Could you check a few things on this model? Use its own coordinates, in mm. A direction names the side the tool comes from. Coordinates: 2 decimals unless noted, no trailing zeros. Loops run counter-clockwise (first coordinate to the right, second up) from the corner with the lowest first, then second, coordinate; pieces in that order, holes last.
from build123d import *

# Parameters (mm, degrees)
SKETCH_1_R          = 12.5
EXTRUDE_3_DEPTH     = 30
SKETCH_3_R          = 1.5
CUT_EXTRUDE_1_DEPTH = 15
SKETCH_4_R          = 6
EXTRUDE_4_DEPTH     = 2
SKETCH_5_R          = 2
EXTRUDE_5_DEPTH     = 10


with BuildPart() as part:
    # 草图1 → 凸台-拉伸3 (new body)
    with BuildSketch(Plane.XY):
        Circle(SKETCH_1_R)
    extrude(amount=EXTRUDE_3_DEPTH)

    # 草图3 → 切除-拉伸1 (cut)
    with BuildSketch(Plane(origin=(0, 0, 0), x_dir=(-1, 0, 0), z_dir=(0, 0, -1))):
        with Locations((8.5, 0)):
            Circle(SKETCH_3_R)
        with Locations((-8.5, 0)):
            Circle(SKETCH_3_R)
    extrude(amount=-CUT_EXTRUDE_1_DEPTH, mode=Mode.SUBTRACT)

    # 草图4 → 凸台-拉伸4 (add)
    with BuildSketch(Plane(origin=(0, 0, 0), x_dir=(-1, 0, 0), z_dir=(0, 0, -1))):
        with Locations(Location((0, 0, 0), (0, 0, 180))):
            Circle(SKETCH_4_R)
    extrude(amount=EXTRUDE_4_DEPTH)

    # 草图5 → 凸台-拉伸5 (add)
    with BuildSketch(Plane(origin=(0, 0, -2), x_dir=(-1, 0, 0), z_dir=(0, 0, -1))):
        Circle(SKETCH_5_R)
    extrude(amount=EXTRUDE_5_DEPTH)


solid = part.part
1) We'd pull the mould along X, two halves only. Please class faces 3 (the flat face through (-3, -5.4, 0)), 4 (the cylindrical face through (5.723, -1.802, -0.986)), 5 (the cylindrical face through (-7.3, -0.9, 7.4)): released by +X, released by -X, zero draft, split by the parting line, or undercut.
2) Imagine slicing it at A-A on y = 0. List the corners of the cut face in (x, z) for me, plus the area to 3 significant figures.
3) Imagine slicing it at D-D on z = 20. List the corners of the cut face in (x, y) for me.
4) Will these pins go through, and if not, where does the flat tip stop? pin 1 (4 mm diameter, centred on x = 8.5, y = 0, fed in from -Z); pin 2 (6 mm diameter, centred on x = -8, z = 17, fed in from -Y); pin 3 (5 mm diameter, centred on y = 6, z = 22, fed in from +X).
5) Imagine slicing it at B-B on x = 0. List the corners of the cut face in (y, z) for me.
6) If I drill on L1, parallel to Z at x = 8.5, y = -6.5; L2, parallel to Y at x = 8.5, z = 7.25; L3, parallel to Z at x = -3, y = -2.5, over which ranges is the centre line in solid material (lowest first)?
7) For faces 1 (the cylindrical face through (10, 0, 7)), 2 (the flat face through (0, 0, -12)), which set-ups out of +Z, -Z, +X, -X, +Y, -Y let a thin tool reach every point of the face, with its end or its side?
8) Imagine slicing it at C-C on z = 7. List the corners of the cut face in (x, y) for me.
Solved:
1. face 3: zero draft
1. face 4: split by the parting line
1. face 5: undercut
2. outline: (-12.5, 0) - (-10, 0) - (-10, 15) - (-7, 15) - (-7, 0) - (-6, 0) - (-6, -2) - (-2, -2) - (-2, -12) - (2, -12) - (2, -2) - (6, -2) - (6, 0) - (7, 0) - (7, 15) - (10, 15) - (10, 0) - (12.5, 0) - (12.5, 30) - (-12.5, 30) - close
2. area: 724 mm2
3. outline: circle Ø25 at (0, 0)
4. pin 1: stops at z = 0
4. pin 2: stops at y = -11.46
4. pin 3: stops at x = 12
5. outline: (-12.5, 0) - (-6, 0) - (-6, -2) - (-2, -2) - (-2, -12) - (2, -12) - (2, -2) - (6, -2) - (6, 0) - (12.5, 0) - (12.5, 30) - (-12.5, 30) - close
6. L1: z = 0 to 30
6. L2: y = -9.17 to -1.5, 1.5 to 9.17
6. L3: z = -2 to 30
7. face 1: -Z
7. face 2: -Z, +X, -X, +Y, -Y
8. outline: circle Ø25 at (0, 0); hole circle Ø3 at (-8.5, 0); hole circle Ø3 at (8.5, 0)
